```python
from build123d import *

# Parameters (mm, degrees)
F0_W           = 584.2
F0_H           = 203.2
F1_DEPTH       = 9.525
F3_D           = 3.6576
F3_DEPTH       = 10.3124
F3_CSINK_D     = 7.7978
F3_CSINK_ANGLE = 82
F3_TIP         = 1.0988539001
F4_W           = 101.6
F4_H           = 69.85
F5_DEPTH       = 9.526
F6_DEPTH       = 25.4
F9_D           = 2.7051
F9_DEPTH       = 13.4874
F9_TIP         = 0.8126940303
F9_ON_F7_D     = 2.7051
F9_ON_F7_DEPTH = 13.4874
F9_ON_F7_TIP   = 0.8126940303


# Not quite as in the source:
# - a feature names something its author has since deleted; it is built from what else it names


with BuildPart() as f1:
    # F0 (on Front) → F1 (new body)
    with BuildSketch(Plane.XZ):
        with Locations((-292.1, 101.6)):
            Rectangle(F0_W, F0_H)
    extrude(amount=F1_DEPTH)

    # F3
    with Locations(Plane.XZ.offset(9.525)):
        with Locations((-238.76, 6.35), (-25.4, 6.35), (-345.44, 6.35), (-558.8, 6.35), (-132.08, 6.35), (-452.12, 6.35), (-152.75, 99.05), (-152.75, 35.05), (-38.75, 25.05), (-14.75, 99.05)):
            CounterSinkHole(F3_D / 2, F3_CSINK_D / 2, depth=F3_DEPTH, counter_sink_angle=F3_CSINK_ANGLE)
            with Locations((0, 0, -(F3_DEPTH + F3_TIP / 2))):  # 118° drill point
                Cone(0, F3_D / 2, F3_TIP, mode=Mode.SUBTRACT)

    # F4 (on face) → F5 (cut, through all)
    with BuildSketch(Plane.XZ.offset(9.525)):
        with Locations((-76.2, 66.675)):
            Rectangle(F4_W, F4_H)
    extrude(amount=-F5_DEPTH, mode=Mode.SUBTRACT)

    # F2 (on face) → F6 (cut)
    with BuildSketch(Plane.XZ.offset(9.525)):
        with BuildLine():
            Line((-30.975, 105.05), (-136.525, 105.05))
            ThreePointArc((-136.525, 105.05), (-141.0151280605, 103.1901280605), (-142.875, 98.7))
            Line((-142.875, 98.7), (-142.875, 95.525))
            ThreePointArc((-142.875, 95.525), (-144.7348719395, 91.0348719395), (-149.225, 89.175))
            Line((-149.225, 89.175), (-152.4, 89.175))
            ThreePointArc((-152.4, 89.175), (-156.8901280605, 87.3151280605), (-158.75, 82.825))
            Line((-158.75, 82.825), (-158.75, 50.8))
            ThreePointArc((-158.75, 50.8), (-156.8901280605, 46.3098719395), (-152.4, 44.45))
            Line((-152.4, 44.45), (-149.225, 44.45))
            ThreePointArc((-149.225, 44.45), (-144.7348719395, 42.5901280605), (-142.875, 38.1))
            Line((-142.875, 38.1), (-142.875, 25.4))
            ThreePointArc((-142.875, 25.4), (-141.0151280605, 20.9098719395), (-136.525, 19.05))
            Line((-136.525, 19.05), (-56.375, 19.05))
            ThreePointArc((-56.375, 19.05), (-51.8848719395, 20.9098719395), (-50.025, 25.4))
            ThreePointArc((-50.025, 25.4), (-48.1651280605, 29.8901280605), (-43.675, 31.75))
            Line((-43.675, 31.75), (-15.1, 31.75))
            ThreePointArc((-15.1, 31.75), (-10.6098719395, 33.6098719395), (-8.75, 38.1))
            Line((-8.75, 38.1), (-8.75, 82.825))
            ThreePointArc((-8.75, 82.825), (-10.6098719395, 87.3151280605), (-15.1, 89.175))
            Line((-15.1, 89.175), (-18.275, 89.175))
            ThreePointArc((-18.275, 89.175), (-22.7651280605, 91.0348719395), (-24.625, 95.525))
            Line((-24.625, 95.525), (-24.625, 98.7))
            ThreePointArc((-24.625, 98.7), (-26.4848719395, 103.1901280605), (-30.975, 105.05))
        make_face()
    extrude(amount=-F6_DEPTH, mode=Mode.SUBTRACT)

    # F9
    with Locations(Plane.YZ):
        with Locations((-4.7625, 184.15), (-4.7625, 101.6), (-4.7625, 19.05)):
            Hole(F9_D / 2, depth=F9_DEPTH)
            with Locations((0, 0, -(F9_DEPTH + F9_TIP / 2))):  # 118° drill point
                Cone(0, F9_D / 2, F9_TIP, mode=Mode.SUBTRACT)

    # F9 on F7
    with Locations(Plane(origin=(-584.2, 0, 0), x_dir=(0, -1, 0), z_dir=(-1, 0, 0))):
        with Locations((4.7625, 184.15), (4.7625, 101.6), (4.7625, 19.05)):
            Hole(F9_ON_F7_D / 2, depth=F9_ON_F7_DEPTH)
            with Locations((0, 0, -(F9_ON_F7_DEPTH + F9_ON_F7_TIP / 2))):  # 118° drill point
                Cone(0, F9_ON_F7_D / 2, F9_ON_F7_TIP, mode=Mode.SUBTRACT)


solid = f1.part
```
The listing builds one solid part. Answer for the finished solid, in the listing's coordinates (mm). A direction names the side the tool comes from. Give positions to 0.01 mm unless a question says otherwise; leave off trailing zeros. Order: outer loops, then holes, each group sorted by start corner. A loop starts at its lowest first (then second) coordinate and runs counter-clockwise, first axis right, second up. Notation, with made-up numbers: M 39,29.25 L 59,29.25 A25 ccw 59,41.25 Z; hole C -34,54.25 d5. An arc over 180 degrees is marked long. Put each result on its own line as item: value. Start each with the question number.
Item 1: Find the intervals of material crossed by line 1 along X through (y, z) = (-5, 99.05); line 2 along Z through (x, y) = (-83.5, -0.75); line 3 along Z through (x, y) = (-132.08, -4), in increasing order.
Item 2: For a pull along Z with two mould halves and no side action, classify faces 1 (the face through (-296, -5, 0)), 2 (the face through (-30, -5, 31.75)), 3 (the face through (0, -5, 100)) as +Z half, -Z half, draft (parallel to the pull), parting line (faces both ways), or undercut.
Item 3: Which of the six approach directions +Z, -Z, +X, -X, +Y, -Y give full straight-line access (tool end or side, diameter ignored) to faces 4 (the face through (-83, -5, 105.05)), 5 (the face through (-296, 0, 103))?
Item 4: The part is cut by section A-A, the plane x = -69.5. Determine the outline of the cut face in (y, z) (3 decimals).
Item 5: Flat-ended cylindrical pins translate along their axes: P1, Ø2, axis at x = -152.75, z = 99.05, coming from the +Y side; P2, Ø1.6, axis at y = -4.76, z = 19.05, coming from the +X side; P3, Ø2.5, axis at y = -4.76, z = 19.05, coming from the +X side; P4, Ø5, axis at x = -14.75, z = 99.05, coming from the -Y side. Find the tip coordinate at first contact, or state that the pin passes through.
Answer key:
1. line 1: x = -584.2 to -154.58, -150.92 to -142.87, -24.63 to -16.58, -12.92 to 0
1. line 2: z = 0 to 19.05, 105.05 to 203.2
1. line 3: z = 0 to 4.52, 8.18 to 19.05, 105.05 to 203.2
2. face 1: -Z half
2. face 2: undercut
2. face 3: draft
3. face 4: +Y, -Y
3. face 5: +Z, -Z, +X, -X, +Y
4. outline: M -9.525,0 L 0,0 L 0,19.05 L -9.525,19.05 Z; M -9.525,105.05 L 0,105.05 L 0,203.2 L -9.525,203.2 Z
5. P1: passes through
5. P2: stops at x = -13.82
5. P3: stops at x = -13.55
5. P4: stops at y = -7.92
